Study the drawing (mm; zero at the part's minimum x, y, z) and answer. Give positions to 0.01 mm unless a question says otherwise; leave off trailing zeros. Loops run counter-clockwise (first coordinate to the right, second up) from the corner with the lowest first, then second, coordinate; pieces in that order, holes last. Notation, with made-up numbers: (4.25, -20) -> (42.25, -20) arc R17 ccw to (42.25, -1) -> close; hole circle Ø2 at (57.5, 75.5). An arc over 180 degrees is marked (long way). One line per question, with ' | ' between items. Start each with the question number.
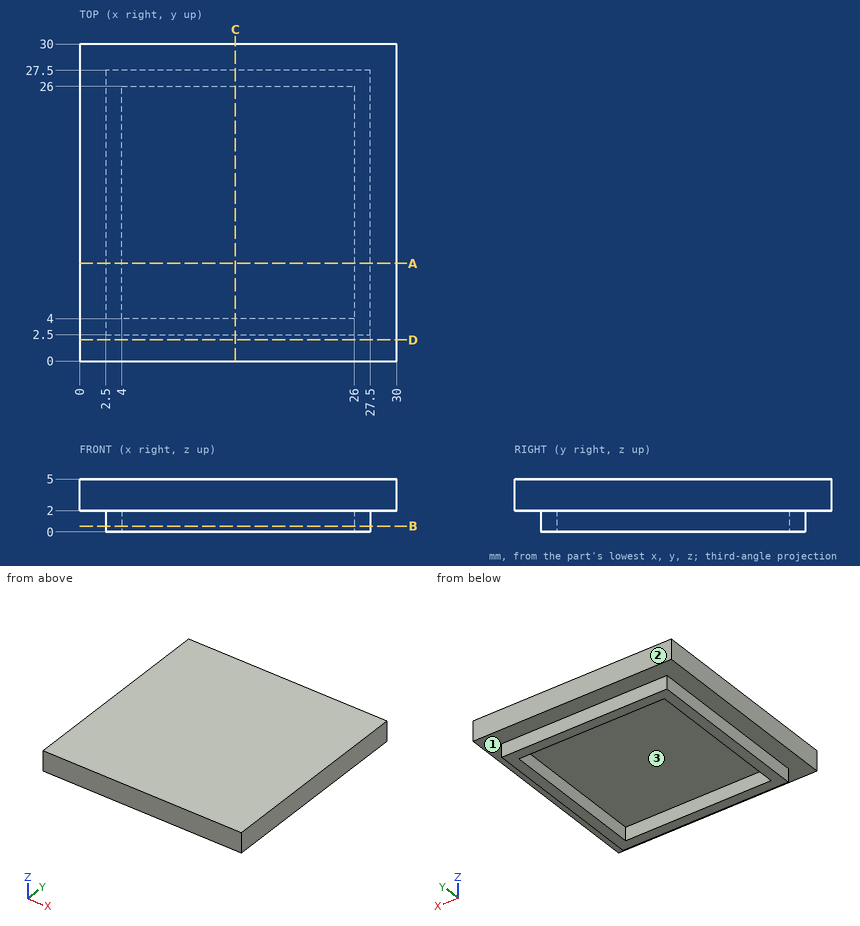
1. Straight lines are drawn through the part: L1, parallel to Y at x = 5.5, z = 1.95; L2, parallel to Z at x = 20, y = 11.5. For each, find the intervals that lie inside material, in ascending order.
2. The part is cut by section D-D (y = 2). Write down the section's boundary in (x, z).
3. Each of these flat-tipped pins is pushed along its axis until it touches: pin 1 Ø1 at (y, z) = (9.5, 1) entering from +X; pin 2 Ø12 at (x, y) = (25, 6.5) entering from -Z; pin 3 Ø0.6 at (x, z) = (16.5, 0.5) entering from -Y; pin 4 Ø5 at (x, y) = (16, 22) entering from -Z. Where does it stop, or does it pass through?
4. Determine the mould class of the marked faces 1, 2 and 3 for opening direction Y: released by +Y, released by -Y, zero draft, split by the parting line, or undercut.
5. The part is cut by section B-B (z = 0.55). Write down the section's boundary in (x, y).
6. The part is cut by section A-A (y = 9.25). Write down the section's boundary in (x, z), plus the area to 3 significant figures.
Check sheet entries:
1) L1: y = 2.5 to 4, 26 to 27.5 | L2: z = 2 to 5
2) outline: (0, 2) -> (30, 2) -> (30, 5) -> (0, 5) -> close
3) pin 1: stops at x = 27.5 | pin 2: stops at z = 0 | pin 3: stops at y = 2.5 | pin 4: stops at z = 2
4) face 1: zero draft | face 2: released by +Y | face 3: undercut
5) outline: (2.5, 2.5) -> (27.5, 2.5) -> (27.5, 27.5) -> (2.5, 27.5) -> close; hole (4, 4) -> (26, 4) -> (26, 26) -> (4, 26) -> close
6) outline: (0, 2) -> (2.5, 2) -> (2.5, 0) -> (4, 0) -> (4, 2) -> (26, 2) -> (26, 0) -> (27.5, 0) -> (27.5, 2) -> (30, 2) -> (30, 5) -> (0, 5) -> close | area: 96.0 mm^2
